Verification items for this drawing (mm, ordinates from the low corner). Give positions to 0.01 mm unless a question says otherwise; leave off trailing zeros. Loops run counter-clockwise (first coordinate to the right, second up) from the corner with the lowest first, then second, coordinate; pieces in that order, holes last. Notation, with made-up numbers: M -29.5,80 L 13.5,80 A20 ccw 13.5,104 Z; hole C 67,-16.75 d10. An arc over 180 degrees is marked long. Use a Markdown table: item, result.
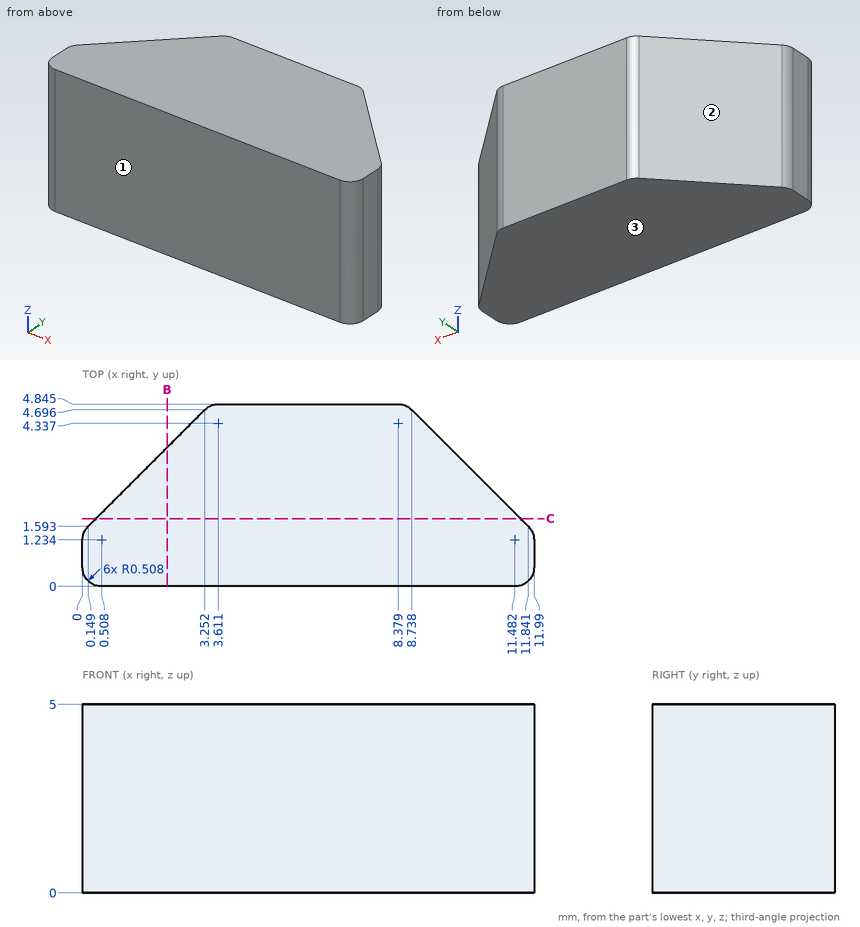
(1) Draft check along Y on the marked faces 1, 2 and 3. Enter one of: +Y half, -Y half, draft (parallel to the pull), parting line (faces both ways), or undercut.
Results below:
| item | result |
|---|---|
| face 1 | -Y half |
| face 2 | +Y half |
| face 3 | draft |
(2) Gauge pin test, flat end, axial feed: P1, Ø1, axis at x = 9.5, z = 4, coming from the +Y side (1 decimal). Record the tip position at first contact, or that the pin passes through.
Results below:
| item | result |
|---|---|
| P1 | y = 4.4 |
(3) Cross-section at B-B on x = 2.25. Record the cut outline in (y, z), then the cut area to 3 significant figures.
Results below:
| item | result |
|---|---|
| outline | M 0,0 L 3.69,0 L 3.69,5 L 0,5 Z |
| area | 18.5 mm^2 |
(4) Cross-section at C-C on y = 1.8. Record the cut outline in (x, z).
Results below:
| item | result |
|---|---|
| outline | M 0.36,0 L 11.63,0 L 11.63,5 L 0.36,5 Z |
(5) Material ranges on line 1 (Y direction, x = 9.25, z = 4.4) (1 decimal); line 2 (X direction, y = 0.35, z = 2.4) (1 decimal); line 3 (X direction, y = 4, z = 4.7) (1 decimal), recorded low to high.
Results below:
| item | result |
|---|---|
| line 1 | 0 to 4.2 |
| line 2 | 0 to 12 |
| line 3 | 2.6 to 9.4 |
